Autodesk Inventor part; units mm, degrees
ref_plane "YZ Plane" through (0, 0, 0) normal (1, 0, 0) x (0, 1, 0)
ref_plane "XZ Plane" through (0, 0, 0) normal (0, 1, 0) x (-1, 0, 0)
ref_plane "XY Plane" through (0, 0, 0) normal (0, 0, 1) x (1, 0, 0)
sketch "Base" plane through (0, 0, 0) normal (0, 0, 1) x (1, 0, 0)
  line L0 (-10, -8) -> (10, -8)
  line L1 (10, -8) -> (10, 8)
  line L2 (10, 8) -> (-10, 8)
  line L3 (-10, 8) -> (-10, -8)
  line L4 (-10, -8) -> (10, 8) construction
  line L5 (10, -8) -> (-10, 8) construction
  point P0 (0, 0)
  dimension "d0" = 20
  dimension "d1" = 16
extrude "Plate1" add sketch "Base" along normal blind 1
sketch "Sketch2" plane through (10, -7, 0) normal (0, -1, 0) x (1, 0, 0)
  line L0 (-20, 0) -> (0, 0)
  line L1 (0, 0) -> (0, 8)
  line L2 (0, 8) -> (-20, 8)
  line L3 (-20, 8) -> (-20, 0)
edge flange "MountFeature" height 8 angle 90 thickness 1 bend radius 1 thickness toward (0, -1, 0) relief tear relief width 1 relief depth 0.5 edges at (0, -8, 1) wall of the first edge with corners at (-10, -7, 0) (10, -7, 0) (10, -7, 8) (-10, -7, 8)
bend "Bend1"
corner "Corner1"
sketch "MountHoles" plane through (0, 0, 0) normal (0, 0, -1) x (-1, 0, 0)
  circle A0 centre (4.85, 4.448) radius 1.15
  circle A1 centre (-4.85, 4.448) radius 1.15
  point P0 (0, 0)
extrude "MountHolesFeature" cut sketch "MountHoles" against normal blind 1
fillet "EdgeFilletsFeature" radius 1 4 edges at (10, 8, 0.5) (-10, 8, 0.5) (-10, -7.5, 8) (10, -7.5, 8)
sketch "ArmMountHoles" plane through (-10, -8, 2) normal (0, -1, 0) x (1, 0, 0)
  line L0 (0, 3) -> (20, 3) construction
  line L1 (10, -3.8) -> (10, 8.8) construction
  circle A0 centre (3, 3) radius 1
  circle A1 centre (17, 3) radius 1
  line L2 (1, 6) -> (19, 6)
  line L3 (20, 0) -> (20, 5)
  line L4 (0, 0) -> (0, 5)
  point P0 (10, -2)
  dimension "d17" = 2
  dimension "d20" = 3
extrude "ArmMountHolesFeature" cut sketch "ArmMountHoles" against normal blind 1
equation "\"d13\" = Thickness"
equation "\"d18\" = Thickness"
equation "\"d2\" = Thickness"
equation "\"d3\" = BendReliefWidth"
equation "\"d4\" = BendReliefDepth"
equation "\"d5\" = MinimumRemnant"
equation "\"d6\" = TransitionRadius"
equation "\"d9\" = BendRadius"
equation "\"d10\" = CornerReliefSize"
equation "\"d11\" = GapSize"
equation "\"d12\" = JacobiRadiusSize"
equation "\"BendRadius\" = Thickness"
equation "\"BendReliefWidth\" = Thickness"
equation "\"BendReliefDepth\" = 0.5 * Thickness"
equation "\"CornerReliefSize\" = 4 * Thickness"
equation "\"MinimumRemnant\" = 2 * Thickness"
equation "\"TransitionRadius\" = BendRadius"
equation "\"JacobiRadiusSize\" = BendRadius"
equation "\"GapSize\" = Thickness"
properties part number "LimitSwitchMount"
Could you check a few things on this model? Use its own coordinates, in mm. A direction names the side the tool comes from. Coordinates: 2 decimals unless noted, no trailing zeros. Loops run counter-clockwise (first coordinate to the right, second up) from the corner with the lowest first, then second, coordinate; pieces in that order, holes last. Notation, with made-up numbers: M 16.25,-28.5 L 43.25,-28.5 A25 cw 43.25,-12.5 Z; hole C 5.25,60 d11. An arc over 180 degrees is marked long. Put each result on its own line as item: value. Start each with the question number.
(1) Suppose I cut it at A-A on x = -4.85. Please give me the cut outline in (y, z), then the cut area to 3 significant figures.
(2) Suppose I cut it at B-B on z = 5. Please give me the cut outline in (x, y), then the cut area to 3 significant figures.
(3) I need wall thicknesses on line 1 (Z direction, x = -4.25, y = -3.25); line 2 (Y direction, x = -0.25, z = 2.5); line 3 (Z direction, x = -7, y = -7.55). Which ranges of each line are inside material? Lowest first, please. Write a range as from..to.
(4) Suppose I cut it at C-C on y = 4.75. Please give me the cut outline in (x, z), then the cut area to 3 significant figures.
(5) For faces 4 (the face through (-9.699, -7.507, 7.715)), 5 (the face through (0, 1, 1)), which set-ups out of +Z, -Z, +X, -X, +Y, -Y let a thin tool reach every point of the face, with its end or its side?
(6) Will these pins go through, and if not, where does the flat tip stop? P1, Ø1, axis at x = -6.5, y = 2, coming from the +Z side; P2, Ø4, axis at x = -3, z = 4, coming from the +Y side.
(7) Thinking about a two-plate mould opening in X: for faces 1 (the face through (9.715, -7.507, 7.699)), 2 (the face through (0, 1, 0)), 3 (the face through (-5.95, 4.79, 0.49)), which applies, pulls with the +X half, pulls with the -X half, needs draft (parallel to the pull), parting line crosses it, or undercut?
(8) Suppose I cut it at D-D on x = 2. Please give me the cut outline in (y, z), then the cut area to 3 significant figures.
Solutions:
1. outline: M -8,2 A2 ccw -6,0 L 3.3,0 L 3.3,1 L -6,1 A1 cw -7,2 L -7,8 L -8,8 Z; M 5.6,0 L 8,0 L 8,1 L 5.6,1 Z
1. area: 20.1 mm2
2. outline: M -10,-8 L -8,-8 L -8,-7 L -10,-7 Z; M -6,-8 L 6,-8 L 6,-7 L -6,-7 Z; M 8,-8 L 10,-8 L 10,-7 L 8,-7 Z
2. area: 16.0 mm2
3. line 1: z = 0..1
3. line 2: y = -8..-7
3. line 3: z = 0.74..4, 6..8
4. outline: M -10,0 L -5.96,0 L -5.96,1 L -10,1 Z; M -3.74,0 L 3.74,0 L 3.74,1 L -3.74,1 Z; M 5.96,0 L 10,0 L 10,1 L 5.96,1 Z
4. area: 15.6 mm2
5. face 4: +Z, -X, +Y, -Y
5. face 5: +Z, +X, -X, +Y
6. P1: stops at z = 1
6. P2: stops at y = -7
7. face 1: pulls with the +X half
7. face 2: needs draft
7. face 3: undercut
8. outline: M -8,2 A2 ccw -6,0 L 8,0 L 8,1 L -6,1 A1 cw -7,2 L -7,8 L -8,8 Z
8. area: 22.4 mm2
